Design review of the part built by this model. Coordinates are the model's own, in mm. A direction names the side the tool comes from. Give positions to 0.01 mm unless a question says otherwise; leave off trailing zeros. Order: outer loops, then holes, each group sorted by start corner. A loop starts at its lowest first (then second) coordinate and runs counter-clockwise, first axis right, second up.
Solid Edge part; units mm, degrees
sketch "Sketch1" plane through (0, 0, 0) normal (0, 0, 1) x (1, 0, 0)
  circle A0 centre (0, 0) radius 1.425
extrude "Protrusion1" add sketch "Sketch1" against normal blind 16
sketch "Sketch2" plane through (0, 0, 0) normal (0, -1, 0) x (1, 0, 0)
  line L0 (-1.425, -2) -> (-2.75, 0)
  line L1 (-2.75, 0) -> (0, 0)
  line L2 (-1.425, -2) -> (-1.425, 0)
revolve "RevolvedProtrusion1" add sketch "Sketch2" angle 360 about axis through (0, 0, 0) along (0, 0, 1) material side at (-2.0458, 0, -0.9724)
sketch "Sketch3" plane through (0, 0, 0) normal (0, 0, 1) x (0, -1, 0)
  line L0 (-3.7678, -0.4) -> (3.7678, -0.4)
  line L1 (3.7678, -0.4) -> (3.7678, 0.4)
  line L2 (3.7678, 0.4) -> (-3.7678, 0.4)
  line L3 (-3.7678, 0.4) -> (-3.7678, -0.4)
extrude "ExtrudedCutout_1" cut sketch "Sketch3" against normal blind 0.5
properties material "Graphite"
1. Machinability: for faces 1 (the face through (-1, 0, 0)), 2 (the face through (-1.13, -0.87, -8.9)), which of the approach directions +Z, -Z, +X, -X, +Y, -Y give a long, thin tool a straight path to every point of the face, cutting with its end or side? Answer none if there is none.
Recorded:
face 1: +Z, +X, -X, +Y, -Y
face 2: -Z
2. Take a section at B-B (x = 0). State the section outline as (y, z) points (3 decimals).
Recorded:
outline: (-2.419, -0.5) - (-1.425, -2) - (-1.425, -16) - (1.425, -16) - (1.425, -2) - (2.419, -0.5) - close
3. Take a section at C-C (z = -7). State the section outline as (x, y) points (3 decimals), then the cut area to 3 significant figures.
Recorded:
outline: circle Ø2.85 at (0, 0)
area: 6.38 mm2
4. For pin 1 (0.9 mm diameter, centred on x = 0, y = 0.5, fed in from +Z); pin 2 (3 mm diameter, centred on y = -1, z = -14, fed in from +X) (3 decimals), all flat-tipped, find the tip position at first contact; note any pin that passes through.
Recorded:
pin 1: stops at z = 0
pin 2: stops at x = 1.425
5. Take a section at A-A (y = 0). State the section outline as (x, z) points (3 decimals), then the cut area to 4 significant figures.
Recorded:
outline: (-2.75, 0) - (-1.425, -2) - (-1.425, -16) - (1.425, -16) - (1.425, -2) - (2.75, 0) - (0.4, 0) - (0.4, -0.5) - (-0.4, -0.5) - (-0.4, 0) - close
area: 47.85 mm2
6. For line 1 along X through (y, z) = (1.35, -0.25); line 2 along Z through (x, y) = (-0.8, -1.4); line 3 along Y through (x, z) = (-0.05, -7.25), list the stretches that pass through material, from the lowest coordinate up.
Recorded:
line 1: x = -2.2 to -0.4, 0.4 to 2.2
line 2: z = -1.72 to 0
line 3: y = -1.42 to 1.42
